Could you check a few things on this model? Use its own coordinates, in mm. A direction names the side the tool comes from. Give positions to 0.01 mm unless a question says otherwise; leave off trailing zeros. Loops run counter-clockwise (first coordinate to the right, second up) from the corner with the lowest first, then second, coordinate; pieces in that order, holes last. Notation, with made-up numbers: M 2,-29.5 L 12,-29.5 A13 cw 12,-5.5 Z; hole C 17,-19 d5. An arc over 180 degrees is marked long. Answer in a Markdown table with one row per item. Add a question column.
1. If we section it at A-A on z = 24: List the corners of the cut face in (x, y) for me, then the cut area to 3 significant figures.
2. I need wall thicknesses on line 1 along Y through (x, z) = (-5, -1); line 2 along Y through (x, z) = (5, -3); line 3 along X through (y, z) = (3, -3.5). Which ranges of each line are inside material? Lowest first, please. Write a range as from..to.
3. Which directions (+Z, -Z, +X, -X, +Y, -Y) give clear straight access to the entire face, cutting with the end or side of a thin tool? Please do faces 4 (the cylindrical face through (-9.09, -22.21, -5.99)), 5 (the flat face through (-22.5, -1.97, -3.94)), 6 (the flat face through (17.3, -14.516, -3.944)), 7 (the cylindrical face through (22.134, 9.279, -5.986)), 8 (the flat face through (-9, -23, -2)).
4. I'm going to push flat-ended pins straight in: pin 1 Ø3.5 at (x, y) = (21.5, 11) entering from +Z; pin 2 Ø3.5 at (x, y) = (-20.5, -9) entering from +Z; pin 3 Ø3 at (x, y) = (-10, 0) entering from -Z. Where does each tip first touch, or does it pass through?
5. Thinking about a two-plate mould opening in X: for faces 1 (the cylindrical face through (-8.119, -19.367, -3.944)), 2 (the conical face through (1.883, -8.479, 22.026)), 3 (the conical face through (-21.46, -9, -7.73)), which applies, released by +X, released by -X, zero draft, split by the parting line, or undercut?
```python
from build123d import *

# Parameters (mm, degrees)
F5_DEPTH  = 8
F6_SIZE   = 1
F10_DEPTH = 25


with BuildPart() as f3:
    # F2 (on Front) → F3 (revolve)
    with BuildSketch(Plane.XZ):
        Polygon((-30.5, 2), (-30.5, 0), (0, 0), (0, 30), align=None)
    revolve(axis=Axis((0, 0, 4.0188357234), (0, 0, -1)))

    # F4 (on face) → F5 (join)
    with BuildSketch(Plane(origin=(0, 0, 0), x_dir=(1, 0, 0), z_dir=(0, 0, -1))):
        with BuildLine():
            Line((1.8302705977, 20.9200886599), (2.0917378259, 23.9086727542))
            ThreePointArc((2.0917378259, 23.9086727542), (0, 24), (-2.0917378259, 23.9086727542))
            Line((-2.0917378259, 23.9086727542), (-1.8302705977, 20.9200886599))
            ThreePointArc((-1.8302705977, 20.9200886599), (0, 21), (1.8302705977, 20.9200886599))
        make_face()
        with BuildLine():
            Line((13.4985398034, 16.0869333055), (15.4269026325, 18.3850666349))
            ThreePointArc((15.4269026325, 18.3850666349), (9.1844023768, 22.1731087803), (2.0917378259, 23.9086727542))
            Line((2.0917378259, 23.9086727542), (1.8302705977, 20.9200886599))
            ThreePointArc((1.8302705977, 20.9200886599), (8.0363520797, 19.4014701827), (13.4985398034, 16.0869333055))
        make_face()
        with BuildLine():
            Line((16.0869333055, 13.4985398034), (18.3850666349, 15.4269026325))
            ThreePointArc((18.3850666349, 15.4269026325), (16.9705627485, 16.9705627485), (15.4269026325, 18.3850666349))
            Line((15.4269026325, 18.3850666349), (13.4985398034, 16.0869333055))
            ThreePointArc((13.4985398034, 16.0869333055), (14.8492424049, 14.8492424049), (16.0869333055, 13.4985398034))
        make_face()
        with BuildLine():
            Line((20.9200886599, 1.8302705977), (23.9086727542, 2.0917378259))
            ThreePointArc((23.9086727542, 2.0917378259), (22.1731087803, 9.1844023768), (18.3850666349, 15.4269026325))
            Line((18.3850666349, 15.4269026325), (16.0869333055, 13.4985398034))
            ThreePointArc((16.0869333055, 13.4985398034), (19.4014701827, 8.0363520797), (20.9200886599, 1.8302705977))
        make_face()
        with BuildLine():
            ThreePointArc((23.9086727542, -2.0917378259), (23.977157318, -1.0468652968), (24, 0))
            ThreePointArc((24, 0), (23.977157318, 1.0468652968), (23.9086727542, 2.0917378259))
            Line((23.9086727542, 2.0917378259), (20.9200886599, 1.8302705977))
            ThreePointArc((20.9200886599, 1.8302705977), (20.9800126532, 0.9160071347), (21, 0))
            ThreePointArc((21, 0), (20.9800126532, -0.9160071347), (20.9200886599, -1.8302705977))
            Line((20.9200886599, -1.8302705977), (23.9086727542, -2.0917378259))
        make_face()
        with BuildLine():
            ThreePointArc((18.3850666349, -15.4269026325), (22.1731087803, -9.1844023768), (23.9086727542, -2.0917378259))
            Line((23.9086727542, -2.0917378259), (20.9200886599, -1.8302705977))
            ThreePointArc((20.9200886599, -1.8302705977), (19.4014701827, -8.0363520797), (16.0869333055, -13.4985398034))
            Line((16.0869333055, -13.4985398034), (18.3850666349, -15.4269026325))
        make_face()
        with BuildLine():
            ThreePointArc((15.4269026325, -18.3850666349), (16.9705627485, -16.9705627485), (18.3850666349, -15.4269026325))
            Line((18.3850666349, -15.4269026325), (16.0869333055, -13.4985398034))
            ThreePointArc((16.0869333055, -13.4985398034), (14.8492424049, -14.8492424049), (13.4985398034, -16.0869333055))
            Line((13.4985398034, -16.0869333055), (15.4269026325, -18.3850666349))
        make_face()
        with BuildLine():
            ThreePointArc((2.0917378259, -23.9086727542), (9.1844023768, -22.1731087803), (15.4269026325, -18.3850666349))
            Line((15.4269026325, -18.3850666349), (13.4985398034, -16.0869333055))
            ThreePointArc((13.4985398034, -16.0869333055), (8.0363520797, -19.4014701827), (1.8302705977, -20.9200886599))
            Line((1.8302705977, -20.9200886599), (2.0917378259, -23.9086727542))
        make_face()
        with BuildLine():
            ThreePointArc((-2.0917378259, -23.9086727542), (0, -24), (2.0917378259, -23.9086727542))
            Line((2.0917378259, -23.9086727542), (1.8302705977, -20.9200886599))
            ThreePointArc((1.8302705977, -20.9200886599), (0, -21), (-1.8302705977, -20.9200886599))
            Line((-1.8302705977, -20.9200886599), (-2.0917378259, -23.9086727542))
        make_face()
        with BuildLine():
            ThreePointArc((-15.4269026325, -18.3850666349), (-9.1844023768, -22.1731087803), (-2.0917378259, -23.9086727542))
            Line((-2.0917378259, -23.9086727542), (-1.8302705977, -20.9200886599))
            ThreePointArc((-1.8302705977, -20.9200886599), (-8.0363520797, -19.4014701827), (-13.4985398034, -16.0869333055))
            Line((-13.4985398034, -16.0869333055), (-15.4269026325, -18.3850666349))
        make_face()
        with BuildLine():
            ThreePointArc((-18.3850666349, -15.4269026325), (-16.9705627485, -16.9705627485), (-15.4269026325, -18.3850666349))
            Line((-15.4269026325, -18.3850666349), (-13.4985398034, -16.0869333055))
            ThreePointArc((-13.4985398034, -16.0869333055), (-14.8492424049, -14.8492424049), (-16.0869333055, -13.4985398034))
            Line((-16.0869333055, -13.4985398034), (-18.3850666349, -15.4269026325))
        make_face()
        with BuildLine():
            ThreePointArc((-23.9086727542, -2.0917378259), (-22.1731087803, -9.1844023768), (-18.3850666349, -15.4269026325))
            Line((-18.3850666349, -15.4269026325), (-16.0869333055, -13.4985398034))
            ThreePointArc((-16.0869333055, -13.4985398034), (-19.4014701827, -8.0363520797), (-20.9200886599, -1.8302705977))
            Line((-20.9200886599, -1.8302705977), (-23.9086727542, -2.0917378259))
        make_face()
        with BuildLine():
            Line((-20.9200886599, 1.8302705977), (-23.9086727542, 2.0917378259))
            ThreePointArc((-23.9086727542, 2.0917378259), (-24, 0), (-23.9086727542, -2.0917378259))
            Line((-23.9086727542, -2.0917378259), (-20.9200886599, -1.8302705977))
            ThreePointArc((-20.9200886599, -1.8302705977), (-21, 0), (-20.9200886599, 1.8302705977))
        make_face()
        with BuildLine():
            Line((-16.0869333055, 13.4985398034), (-18.3850666349, 15.4269026325))
            ThreePointArc((-18.3850666349, 15.4269026325), (-22.1731087803, 9.1844023768), (-23.9086727542, 2.0917378259))
            Line((-23.9086727542, 2.0917378259), (-20.9200886599, 1.8302705977))
            ThreePointArc((-20.9200886599, 1.8302705977), (-19.4014701827, 8.0363520797), (-16.0869333055, 13.4985398034))
        make_face()
        with BuildLine():
            Line((-13.4985398034, 16.0869333055), (-15.4269026325, 18.3850666349))
            ThreePointArc((-15.4269026325, 18.3850666349), (-16.9705627485, 16.9705627485), (-18.3850666349, 15.4269026325))
            Line((-18.3850666349, 15.4269026325), (-16.0869333055, 13.4985398034))
            ThreePointArc((-16.0869333055, 13.4985398034), (-14.8492424049, 14.8492424049), (-13.4985398034, 16.0869333055))
        make_face()
        with BuildLine():
            Line((-1.8302705977, 20.9200886599), (-2.0917378259, 23.9086727542))
            ThreePointArc((-2.0917378259, 23.9086727542), (-9.1844023768, 22.1731087803), (-15.4269026325, 18.3850666349))
            Line((-15.4269026325, 18.3850666349), (-13.4985398034, 16.0869333055))
            ThreePointArc((-13.4985398034, 16.0869333055), (-8.0363520797, 19.4014701827), (-1.8302705977, 20.9200886599))
        make_face()
    extrude(amount=F5_DEPTH)

    # F6
    f6_edges = [f3.edges().sort_by_distance(p)[0] for p in [
        (2.091738, 23.908673, -8),
    ]]
    chamfer(f6_edges, length=F6_SIZE)

    # F7 (on Right) → F8 (revolve)
    with BuildSketch(Plane.YZ):
        Polygon((25, -2), (24, -2), (24, -5), align=None)
    revolve(axis=Axis((0, 0, 4.0188357234), (0, 0, -1)))

    # F9 (on Top) + F4 (on face) → F10 (cut)
    with BuildSketch(Plane.XY):
        with BuildLine():
            Line((-23.3643555151, 19.6050220954), (0, 0))
            Line((0, 0), (-19.6050220954, 23.3643555151))
            ThreePointArc((-19.6050220954, 23.3643555151), (-21.5667568262, 21.5667568262), (-23.3643555151, 19.6050220954))
        make_face()
        with BuildLine():
            Line((0, 0), (-30.3839382918, 2.6582501538))
            ThreePointArc((-30.3839382918, 2.6582501538), (-30.5, 0), (-30.3839382918, -2.6582501538))
            Line((-30.3839382918, -2.6582501538), (0, 0))
        make_face()
        with BuildLine():
            Line((-19.6050220954, -23.3643555151), (0, 0))
            Line((0, 0), (-23.3643555151, -19.6050220954))
            ThreePointArc((-23.3643555151, -19.6050220954), (-21.5667568262, -21.5667568262), (-19.6050220954, -23.3643555151))
        make_face()
        with BuildLine():
            Line((2.6582501538, -30.3839382918), (0, 0))
            Line((0, 0), (-2.6582501538, -30.3839382918))
            ThreePointArc((-2.6582501538, -30.3839382918), (0, -30.5), (2.6582501538, -30.3839382918))
        make_face()
        with BuildLine():
            Line((23.3643555151, -19.6050220954), (0, 0))
            Line((0, 0), (19.6050220954, -23.3643555151))
            ThreePointArc((19.6050220954, -23.3643555151), (21.5667568262, -21.5667568262), (23.3643555151, -19.6050220954))
        make_face()
        with BuildLine():
            Line((30.3839382918, 2.6582501538), (0, 0))
            Line((0, 0), (30.3839382918, -2.6582501538))
            ThreePointArc((30.3839382918, -2.6582501538), (30.4709707582, -1.3303913146), (30.5, 0))
            ThreePointArc((30.5, 0), (30.4709707582, 1.3303913146), (30.3839382918, 2.6582501538))
        make_face()
        with BuildLine():
            Line((-2.6582501538, 30.3839382918), (0, 0))
            Line((0, 0), (2.6582501538, 30.3839382918))
            ThreePointArc((2.6582501538, 30.3839382918), (0, 30.5), (-2.6582501538, 30.3839382918))
        make_face()
        with BuildLine():
            Line((19.6050220954, 23.3643555151), (0, 0))
            Line((0, 0), (23.3643555151, 19.6050220954))
            ThreePointArc((23.3643555151, 19.6050220954), (21.5667568262, 21.5667568262), (19.6050220954, 23.3643555151))
        make_face()
    with BuildSketch(Plane(origin=(0, 0, 0), x_dir=(1, 0, 0), z_dir=(0, 0, -1))):
        with BuildLine():
            ThreePointArc((-2.0917378259, 23.9086727542), (0, 24), (2.0917378259, 23.9086727542))
            Line((2.0917378259, 23.9086727542), (2.6582501538, 30.3839382918))
            ThreePointArc((2.6582501538, 30.3839382918), (0, 30.5), (-2.6582501538, 30.3839382918))
            Line((-2.6582501538, 30.3839382918), (-2.0917378259, 23.9086727542))
        make_face()
        with BuildLine():
            Line((23.3643555151, -19.6050220954), (18.3850666349, -15.4269026325))
            ThreePointArc((18.3850666349, -15.4269026325), (16.9705627485, -16.9705627485), (15.4269026325, -18.3850666349))
            Line((15.4269026325, -18.3850666349), (19.6050220954, -23.3643555151))
            ThreePointArc((19.6050220954, -23.3643555151), (21.5667568262, -21.5667568262), (23.3643555151, -19.6050220954))
        make_face()
    extrude(amount=-F10_DEPTH, dir=(0, 0, 1), mode=Mode.SUBTRACT)


solid = f3.part
```
Results:
| question | item | result |
|---|---|---|
| 1 | outline | C 0,0 d13.07 |
| 1 | area | 134 mm2 |
| 2 | line 1 | -23.47..-20.4, 20.4..23.47 |
| 2 | line 2 | -24.15..-20.4, 20.4..24.15 |
| 2 | line 3 | -24.32..-20.78, 20.78..24.32 |
| 3 | face 4 | -Z, -X, -Y |
| 3 | face 5 | -Z, -X |
| 3 | face 6 | -Z, -Y |
| 3 | face 7 | -Z, +X, +Y |
| 3 | face 8 | -X, -Y |
| 4 | pin 1 | z = 9.44 |
| 4 | pin 2 | z = 11.05 |
| 4 | pin 3 | z = 0 |
| 5 | face 1 | undercut |
| 5 | face 2 | split by the parting line |
| 5 | face 3 | released by -X |
